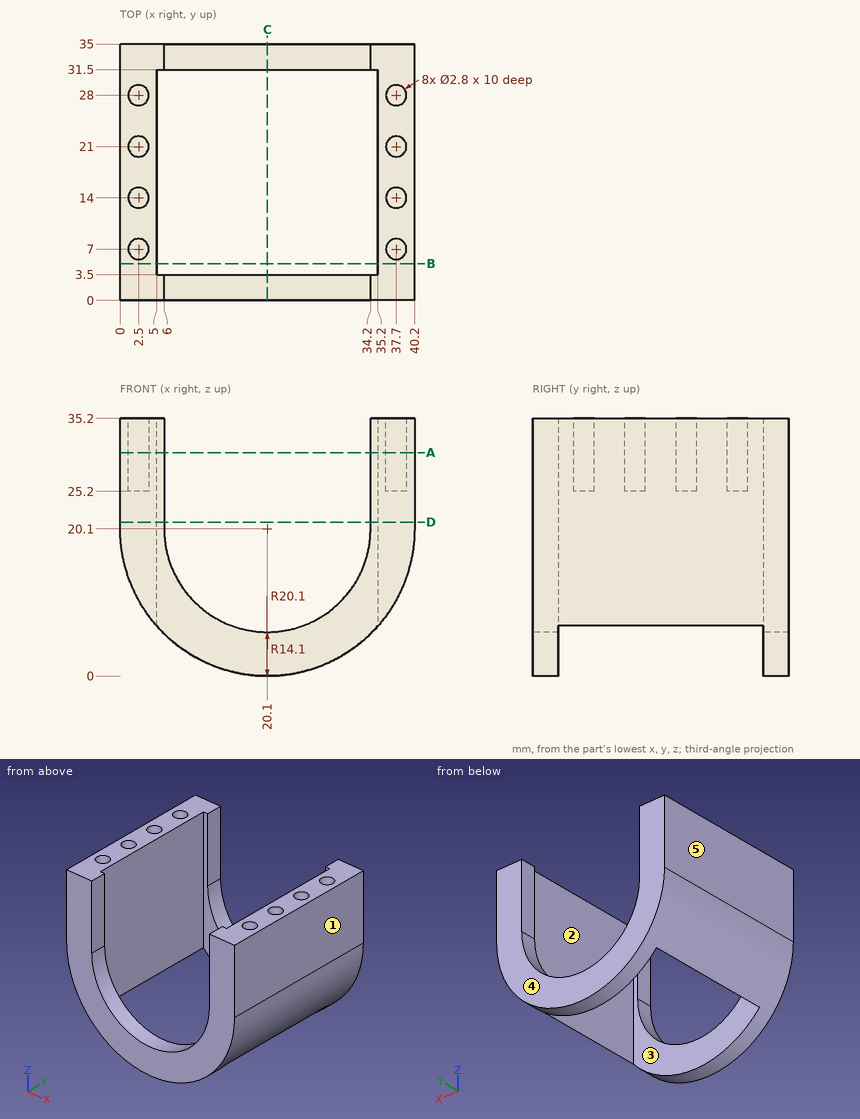
Here's the drawing with two shaded views (mm, measured from the low corner). I have some questions. A direction names the side the tool comes from. Coordinates: 2 decimals unless noted, no trailing zeros. Order: outer loops, then holes, each group sorted by start corner. A loop starts at its lowest first (then second) coordinate and runs counter-clockwise, first axis right, second up.
Item 1: Thinking about a two-plate mould opening in Y: for the marked faces 3, 4 and 5, which applies, pulls with the +Y half, pulls with the -Y half, needs draft (parallel to the pull), parting line crosses it, or undercut?
Response values:
face 3: undercut
face 4: pulls with the +Y half
face 5: needs draft
Item 2: If we section it at A-A, the plane z = 30.5: Give the number of separate pieces and of enclosed holes in the cut face, then the cut area to 3 significant figures.
Response values:
separate pieces: 2
enclosed holes: 8
area: 315 mm2
Item 3: I need wall thicknesses on probe 1 along Y at (x, z) = (2.5, 30); probe 2 along Y at (x, z) = (37, 29); probe 3 along X at (y, z) = (28.5, 26.5). Which ranges of each line are inside material? Lowest first, please.
Response values:
probe 1: y = 0 to 5.6, 8.4 to 12.6, 15.4 to 19.6, 22.4 to 26.6, 29.4 to 35
probe 2: y = 0 to 5.79, 8.21 to 12.79, 15.21 to 19.79, 22.21 to 26.79, 29.21 to 35
probe 3: x = 0 to 1.19, 3.81 to 5, 35.2 to 36.39, 39.01 to 40.2
Item 4: If we section it at B-B, the plane y = 5: List the corners of the cut face in (x, z) for me.
Response values:
outline: (0, 20.1) arc R20.1 ccw to (5, 6.83) - (5, 35.2) - (0, 35.2) - close; (35.2, 6.83) arc R20.1 ccw to (40.2, 20.1) - (40.2, 35.2) - (35.2, 35.2) - close
Item 5: I'm going to push flat-ended pins straight in: pin 1 Ø2.5 at (x, y) = (37.7, 28) entering from -Z; pin 2 Ø2 at (x, y) = (7.5, 12.5) entering from -Z; pin 3 Ø4.5 at (x, y) = (2.5, 14) entering from -Z; pin 4 Ø3.5 at (x, y) = (37.7, 7) entering from -Z. Where does each tip first touch, or does it pass through?
Response values:
pin 1: stops at z = 8.41
pin 2: passes through
pin 3: stops at z = 7.12
pin 4: stops at z = 7.74
Item 6: If we section it at D-D, the plane z = 21: List the corners of the cut face in (x, y) for me, then the cut area to 3 significant figures.
Response values:
outline: (0, 0) - (6, 0) - (6, 3.5) - (5, 3.5) - (5, 31.5) - (6, 31.5) - (6, 35) - (0, 35) - close; (34.2, 0) - (40.2, 0) - (40.2, 35) - (34.2, 35) - (34.2, 31.5) - (35.2, 31.5) - (35.2, 3.5) - (34.2, 3.5) - close
area: 364 mm2
Item 7: Which directions (+Z, -Z, +X, -X, +Y, -Y) give clear straight access to the entire face, cutting with the end or side of a thin tool? Please do the marked faces 1 and 2.
Response values:
face 1: +Z, -Z, +X, +Y, -Y
face 2: +Z, -Z
Item 8: If we section it at C-C, the plane x = 20.1: List the corners of the cut face in (y, z) for me.
Response values:
outline: (0, 0) - (3.5, 0) - (3.5, 6) - (0, 6) - close; (31.5, 0) - (35, 0) - (35, 6) - (31.5, 6) - close
